Autodesk Fusion 360 part; units mm, degrees
sketch "Skizze1" plane through (0, 0, 0) normal (0, 1, 0) x (1, 0, 0)
  line L0 (0, 0) -> (258, 0)
  line L1 (258, 0) -> (258, 237)
  line L2 (0, 0) -> (0, 185)
  line L3 (0, 185) -> (258, 185)
  line L4 (258, 237) -> (0, 237)
  line L5 (0, 237) -> (0, 185)
  line L6 (0, 185) -> (24.5, 185)
  line L7 (258, 185) -> (233.5, 185)
  line L8 (24.5, 237) -> (233.5, 237)
  line L9 (0, 185) -> (24.5, 237)
  line L10 (258, 185) -> (233.5, 237)
  dimension "d1" = 258
  dimension "d2" = 237
  dimension "d3" = 185
  dimension "d4" = 24.5
  dimension "d5" = 24.5
  dimension "d6" = 209
extrude "Extrusion1" add sketch "Skizze1" along normal blind 5 contours L0 L1 L2 L3 L6 L7 | L3 L4 L6 L7 L8 L9 L10
sketch "Skizze2" plane through (0, 5, 0) normal (0, 1, 0) x (-1, 0, 0)
  line L0 (0, 0) -> (-258, 0)
  line L1 (-258, 0) -> (-258, -185)
  line L2 (-258, -185) -> (-233.5, -237)
  line L3 (-233.5, -237) -> (-24.5, -237)
  line L4 (-24.5, -237) -> (0, -185)
  line L5 (0, -185) -> (0, 0)
  line L6 (0, -185) -> (-258, -185)
  line L7 (0, 0) -> (0, -125)
  line L8 (0, -125) -> (-22, -125)
  line L9 (-22, -125) -> (-129, -125)
  line L10 (-129, -125) -> (-129, -178)
  line L11 (-129, -178) -> (-22, -178)
  line L12 (-22, -178) -> (-22, -125)
  dimension "d9" = 125
  dimension "d10" = 22
  dimension "d11" = 107
  dimension "d12" = 53
extrude "Extrusion2" cut sketch "Skizze2" against normal blind 50 contours L9 L10 L11 L12
sketch "Skizze3" plane through (0, 5, 0) normal (0, 1, 0) x (-1, 0, 0)
  line L0 (-129, -125) -> (-22, -125)
  line L1 (-22, -125) -> (-22, -178)
  line L2 (-22, -178) -> (-129, -178)
  line L3 (-129, -178) -> (-129, -125)
  line L4 (0, 0) -> (-258, 0)
  line L5 (-258, 0) -> (-258, -185)
  line L6 (-258, -185) -> (-233.5, -237)
  line L7 (-233.5, -237) -> (-24.5, -237)
  line L8 (-24.5, -237) -> (0, -185)
  line L9 (0, -185) -> (0, 0)
  line L10 (0, -185) -> (-30.8644, -237)
  line L11 (-258, -185) -> (-230, -237)
extrude "Extrusion3" cut sketch "Skizze3" against normal blind 30 contours L7 L8 L10 | L6 L7 L11
sketch "Skizze4" plane through (0, 5, 0) normal (0, 1, 0) x (-1, 0, 0)
  line L0 (-30.8644, -237) -> (0, -185)
  line L1 (0, -185) -> (0, 0)
  line L2 (0, 0) -> (-258, 0)
  line L3 (-258, 0) -> (-258, -185)
  line L4 (-258, -185) -> (-230, -237)
  line L5 (-230, -237) -> (-30.8644, -237)
  line L6 (-129, -125) -> (-22, -125)
  line L7 (-22, -125) -> (-22, -178)
  line L8 (-22, -178) -> (-129, -178)
  line L9 (-129, -178) -> (-129, -125)
  line L10 (-30.8644, -237) -> (0, -237)
  line L11 (0, -237) -> (0, -185)
  line L12 (-258, -185) -> (-258, -237)
  line L13 (-258, -237) -> (-230, -237)
extrude "Extrusion4" add sketch "Skizze4" against normal blind 5 contours L0 L10 L11 | L4 L12 L13
sketch "Skizze5" plane through (0, 5, 0) normal (0, 1, 0) x (-1, 0, 0)
  line L0 (0, -237) -> (0, 0)
  line L1 (0, 0) -> (-258, 0)
  line L2 (-258, 0) -> (-258, -237)
  line L3 (-258, -237) -> (-230, -237)
  line L4 (-230, -237) -> (0, -237)
  line L5 (-129, -125) -> (-22, -125)
  line L6 (-22, -125) -> (-22, -178)
  line L7 (-22, -178) -> (-129, -178)
  line L8 (-129, -178) -> (-129, -125)
  line L9 (0, -237) -> (-24, -237)
  line L10 (-258, -237) -> (-234, -237)
  line L11 (0, -237) -> (0, -187)
  line L12 (-258, -237) -> (-258, -187)
  line L13 (0, -187) -> (-24, -237)
  line L14 (-258, -187) -> (-234, -237)
  dimension "d19" = 24
  dimension "d20" = 24
  dimension "d21" = 50
  dimension "d22" = 50
extrude "Extrusion5" cut sketch "Skizze5" against normal blind 45 contours L0 L4 L9 L11 L13 | L2 L3 L10 L12 L14
sketch "Skizze6" plane through (0, 5, 0) normal (0, 1, 0) x (-1, 0, 0)
  line L0 (-24, -237) -> (0, -187)
  line L1 (0, -187) -> (0, 0)
  line L2 (0, 0) -> (-258, 0)
  line L3 (-258, 0) -> (-258, -187)
  line L4 (-258, -187) -> (-234, -237)
  line L5 (-234, -237) -> (-230, -237)
  line L6 (-230, -237) -> (-24, -237)
  line L7 (-129, -125) -> (-22, -125)
  line L8 (-22, -125) -> (-22, -178)
  line L9 (-22, -178) -> (-129, -178)
  line L10 (-129, -178) -> (-129, -125)
  line L11 (0, 0) -> (0, -195)
  line L12 (-258, 0) -> (-258, -195)
  line L13 (0, -195) -> (-24, -237)
  line L14 (-258, -195) -> (-234, -237)
  dimension "d25" = 195
  dimension "d26" = 195
extrude "Extrusion6" add sketch "Skizze6" against normal blind 5 contours L0 L11 L13 | L4 L12 L14
Build history of the part. All positions in model axes, mm. Round coordinates to 2 decimals unless told otherwise and drop trailing zeros. Loops run counter-clockwise (first coordinate to the right, second up) from the corner with the lowest first, then second, coordinate; pieces in that order, holes last. Notation, with made-up numbers: (27, 42) -> (41, 42) arc R36 cw to (41, 79) -> close; hole circle Ø9 at (86, 60.25). An arc over 180 degrees is marked (long way). Answer in a Markdown table with one row per item.
Item 1: Saw through at D-D (z = -216.5). Write the cut outline in (x, y), and give its area (3 significant figures).
Answers below:
| item | result |
|---|---|
| outline | (12.29, 0) -> (245.71, 0) -> (245.71, 5) -> (12.29, 5) -> close |
| area | 1,170 mm² |
Item 2: Saw through at B-B (z = -138.5). Write the cut outline in (x, y).
Answers below:
| item | result |
|---|---|
| outline | (0, 0) -> (22, 0) -> (22, 5) -> (0, 5) -> close; (129, 0) -> (258, 0) -> (258, 5) -> (129, 5) -> close |
Item 3: Saw through at C-C (y = 3). Write the cut outline in (x, z).
Answers below:
| item | result |
|---|---|
| outline | (0, -195) -> (24, -237) -> (234, -237) -> (258, -195) -> (258, 0) -> (0, 0) -> close; hole (22, -178) -> (129, -178) -> (129, -125) -> (22, -125) -> close |
Item 4: Saw through at A-A (x = 36). Write the cut outline in (y, z), and give its area (3 significant figures).
Answers below:
| item | result |
|---|---|
| outline | (0, -237) -> (5, -237) -> (5, -178) -> (0, -178) -> close; (0, -125) -> (5, -125) -> (5, 0) -> (0, 0) -> close |
| area | 920 mm² |
Item 5: Drill centre lines: L1, parallel to Z at x = 106.5, y = 3.9; L2, parallel to X at y = 0.7, z = -148; L3, parallel to X at y = 1.3, z = -199. Where is each one in solid material? Low to high. Write a range as [from, to].
Answers below:
| item | result |
|---|---|
| L1 | z = [-237, -178], [-125, 0] |
| L2 | x = [0, 22], [129, 258] |
| L3 | x = [2.29, 255.71] |
